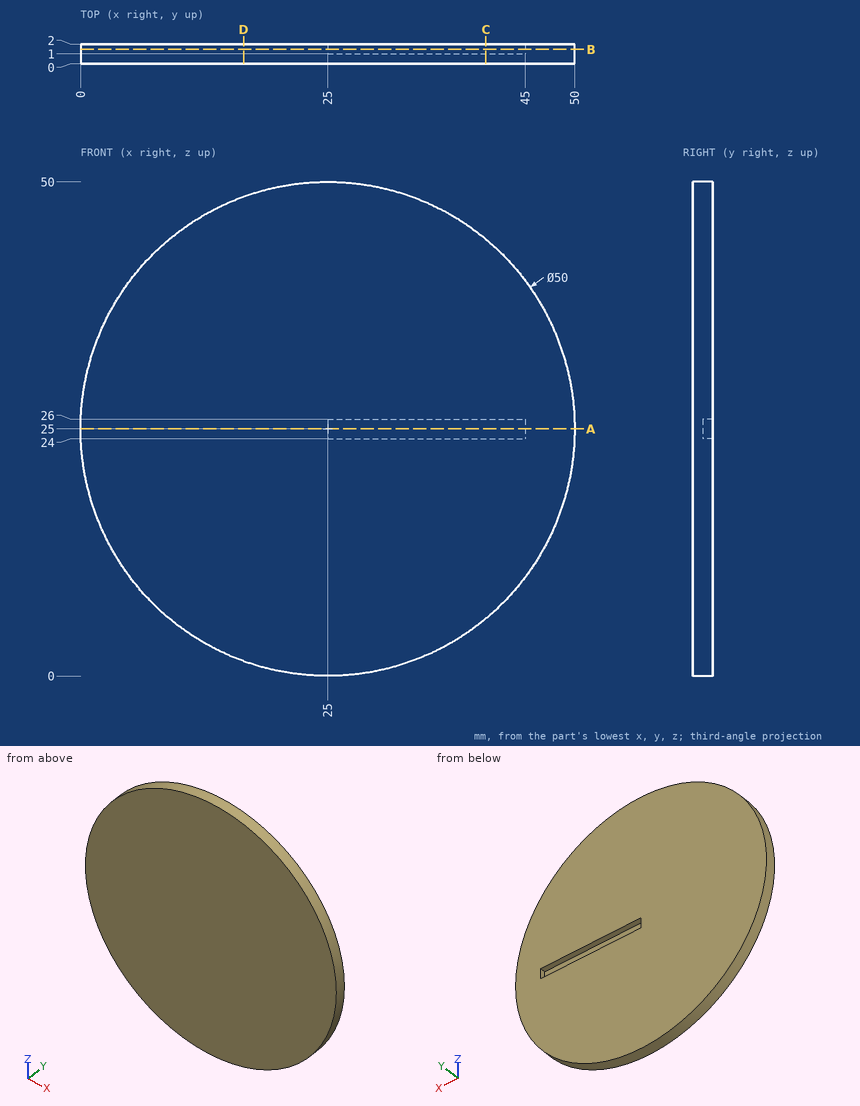
Verification items for this drawing (mm, ordinates from the low corner). Coordinates: 2 decimals unless noted, no trailing zeros. Order: outer loops, then holes, each group sorted by start corner. A loop starts at its lowest first (then second) coordinate and runs counter-clockwise, first axis right, second up. Notation, with made-up numbers: (49, 30) - (81, 30) arc R18 ccw to (81, 57) - close; hole circle Ø9 at (68, -36.75). An arc over 180 degrees is marked (long way). Use one line per item in the form item = value.
1. Gauge pin test, flat end, axial feed: pin 1 (1.1 mm diameter, centred on x = 39, y = 1.5, fed in from +Z). Record the tip position at first contact, or that the pin passes through.
Here are the results:
pin_1 = 46.07
2. Section check C-C (x = 41). Record the boundary of the cut face in (y, z), then the cut area to 3 significant figures.
Here are the results:
outline = (0, 5.79) - (2, 5.79) - (2, 24) - (1, 24) - (1, 26) - (2, 26) - (2, 44.21) - (0, 44.21) - close
area = 74.8 mm²
3. Section check D-D (x = 16.5). Record the boundary of the cut face in (y, z).
Here are the results:
outline = (0, 1.49) - (2, 1.49) - (2, 48.51) - (0, 48.51) - close
4. Section check A-A (z = 25). Record the boundary of the cut face in (x, y).
Here are the results:
outline = (0, 0) - (50, 0) - (50, 2) - (45, 2) - (45, 1) - (25, 1) - (25, 2) - (0, 2) - close
5. Scan lines: line 1 (Z direction, x = 26, y = 1.95); line 2 (Z direction, x = 24, y = 0.6); line 3 (X direction, y = 0.6, z = 10). Record each from-to range of solid material in increasing order.
Here are the results:
line_1 = 0.02 to 24, 26 to 49.98
line_2 = 0.02 to 49.98
line_3 = 5 to 45
6. Section check B-B (y = 1.45). Record the boundary of the cut face in (x, z), then the cut area to 3 significant figures.
Here are the results:
outline = circle Ø50 at (25, 25); hole (25, 24) - (45, 24) - (45, 26) - (25, 26) - close
area = 1,920 mm²
